Read the model definition and answer for the solid it produces. Units are mm, in the model's axes. Face numbers are marked on the shaded views. A direction names the side the tool comes from. Coordinates: 2 decimals unless noted, no trailing zeros. Loops run counter-clockwise (first coordinate to the right, second up) from the corner with the lowest first, then second, coordinate; pieces in that order, holes last.
from build123d import *

# Parameters (mm, degrees)
F1_DEPTH     = 12.7
F0_W         = 50.8
F0_H         = 7.112
F2_DEPTH     = 25.4
F0_W_2       = 12.7
F0_H_2       = 21.59
F3_DEPTH     = 76.2
F4_DEPTH     = 76.2
F5_SIZE2     = 21.9970452561
F5_SIZE      = 12.7
F6_SIZE2     = 21.9970452561
F6_SIZE      = 12.7
F7_R         = 7.62
F8_T1_DEPTH  = 70.3962243683
F8_T3_DEPTH  = 70.3962243683
F8_T5_DEPTH  = 51.8924487366
F8_T7_DEPTH  = 51.8924487366
F8_T13_DEPTH = 89.9924487366
F8_T17_DEPTH = 89.9924487366


# Not quite as in the source:
# - a fillet or chamfer that OpenCascade refuses, or shapes differently, is made with other operations: its cross-section is extruded or revolved along the edge and cut away or added


with BuildPart() as f1:
    # F0 (on Front) → F1 (new body)
    with BuildSketch(Plane.XZ):
        Polygon((25.4, -14.351), (25.4, 7.239), (12.7, 7.239), (-38.1, 7.239), (-38.1, -14.351), align=None)
    extrude(amount=-F1_DEPTH)

    # F0 (on Front) → F2 (join)
    with BuildSketch(Plane.XZ):
        with Locations((-12.7, 10.795)):
            Rectangle(F0_W, F0_H)
    extrude(amount=-F2_DEPTH)

    # F0 (on Front) → F3 (join)
    with BuildSketch(Plane.XZ):
        with Locations((31.75, -3.556)):
            Rectangle(F0_W_2, F0_H_2)
        with Locations((31.75, 10.795)):
            Rectangle(F0_W_2, F0_H)
    extrude(amount=-F3_DEPTH)

    # F0 (on Front) → F4 (join)
    with BuildSketch(Plane.XZ):
        with Locations((19.05, 10.795)):
            Rectangle(F0_W_2, F0_H)
    extrude(amount=-F4_DEPTH)

    # F5
    f5_edges = [f1.edges().sort_by_distance(p)[0] for p in [
        (38.1, 76.2, 0),
    ]]
    f5_side = f1.faces().sort_by_distance((29.228014, 76.2, 2.143688))[0]
    chamfer(f5_edges, length=F5_SIZE, length2=F5_SIZE2, reference=f5_side)

    # F6
    f6_edges = [f1.edges().sort_by_distance(p)[0] for p in [
        (-38.1, 0, 0),
    ]]
    chamfer(f6_edges, length=F6_SIZE, length2=F6_SIZE2)

    # F7
    f7_edges = [f1.edges().sort_by_distance(p)[0] for p in [
        (38.1, 27.101477, 14.351),
        (10.998523, 0, 14.351),
        (38.1, 0, 0),
    ]]
    fillet(f7_edges, radius=F7_R)

    # F8: chamfer of 7.62 on 4 edges, made by hand

    # F8_s2 → F8_t1 (cut)
    with BuildSketch(Plane.YZ.offset(-57.6962243683)):
        Polygon((17.78, 14.351), (25.4, 6.731), (25.4, 14.351), align=None)
    extrude(amount=F8_T1_DEPTH, mode=Mode.SUBTRACT)

    # F8_s4 → F8_t3 (cut)
    with BuildSketch(Plane.XZ.offset(-95.7962243683)):
        Polygon((20.32, 14.351), (12.7, 6.731), (12.7, 14.351), align=None)
    extrude(amount=F8_T3_DEPTH, mode=Mode.SUBTRACT)

    # F8_s6 → F8_t5 (cut)
    with BuildSketch(Plane.YZ.offset(-6.8962243683)):
        Polygon((68.58, 14.351), (76.2, 6.731), (76.2, 14.351), align=None)
    extrude(amount=F8_T5_DEPTH, mode=Mode.SUBTRACT)

    # F8_s8 → F8_t7 (cut)
    with BuildSketch(Plane.XZ.offset(-44.9962243683)):
        Polygon((-30.48, 14.351), (-38.1, 6.731), (-38.1, 14.351), align=None)
    extrude(amount=F8_T7_DEPTH, mode=Mode.SUBTRACT)


with BuildPart() as f8_tool11:
    # F8_s12 → F8_t13 (new body)
    with BuildSketch(Plane.YZ.offset(32.2962243683)):
        Polygon((17.78, 14.351), (25.4, 6.731), (25.4, 14.351), align=None)
    extrude(amount=-F8_T13_DEPTH)

    split(bisect_by=Plane.YZ.offset(12.7), keep=Keep.TOP)


with BuildPart() as f8_tool15:
    # F8_s16 → F8_t17 (new body)
    with BuildSketch(Plane.XZ.offset(-5.8037756317)):
        Polygon((20.32, 14.351), (12.7, 6.731), (12.7, 14.351), align=None)
    extrude(amount=-F8_T17_DEPTH)

    split(bisect_by=Plane.XZ.offset(-25.4), keep=Keep.TOP)


with BuildPart() as f8_tool11_1:
    add(f8_tool11.part)

    # F8_t19: intersect F8_tool15
    add(f8_tool15.part, mode=Mode.INTERSECT)


with BuildPart() as f1_1:
    add(f1.part)

    # F8_t9: cut F8_tool11
    add(f8_tool11_1.part, mode=Mode.SUBTRACT)


solid = f1_1.part
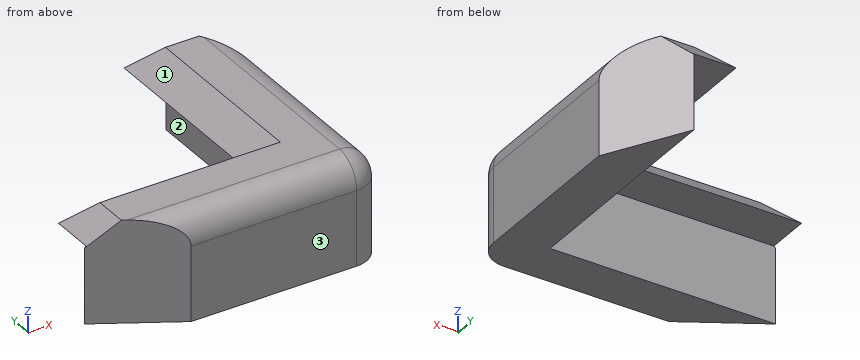
Item 1: Given pin 1 (1.5 mm diameter, centred on y = 63.5, z = 1.5, fed in from -X); pin 2 (6.5 mm diameter, centred on x = 5.5, z = 1, fed in from +Y); pin 3 (12 mm diameter, centred on x = 9.5, y = 41, fed in from +Z), each flat-ended and moving along its own axis, determine where each tip first touches the part or whether it passes through.
Numbers:
pin 1: stops at x = 25.4
pin 2: stops at y = 12.7
pin 3: stops at z = 9.53
Item 2: Which of the six approach directions +Z, -Z, +X, -X, +Y, -Y give full straight-line access (tool end or side, diameter ignored) to the marked faces 1, 2 and 3?
Numbers:
face 1: +Z, -X, +Y
face 2: -Z, -X, +Y
face 3: +Z, -Z, +X, -X, -Y
Item 3: A cutting plane is placed at B-B on z = 3.5. Determine the outline of the cut face in (x, y).
Numbers:
outline: (-38.1, 12.7) - (-16.1, 0) - (30.48, 0) arc R7.62 ccw to (38.1, 7.62) - (38.1, 54.2) - (25.4, 76.2) - (25.4, 12.7) - close
Item 4: A cutting plane is placed at A-A on x = 8. Determine the outline of the cut face in (y, z), then the cut area to 3 significant figures.
Numbers:
outline: (0, -14.35) - (12.7, -14.35) - (12.7, 7.24) - (24.89, 7.24) - (17.78, 14.35) - (7.62, 14.35) arc R7.62 ccw to (0, 6.73) - close
area: 413 mm2
Item 5: Find the intervals of material crossed by line 1 along Y through (x, z) = (2, -11); line 2 along X through (y, z) = (44, 2.75); line 3 along Y through (x, z) = (-18, 5), in increasing order.
Numbers:
line 1: y = 0 to 12.7
line 2: x = 25.4 to 38.1
line 3: y = 1.1 to 12.7
Item 6: A cutting plane is placed at C-C on x = 18. Determine the outline of the cut face in (y, z), then the cut area to 3 significant figures.
Numbers:
outline: (0, -14.35) - (12.7, -14.35) - (12.7, 7.24) - (75.69, 7.24) - (70.9, 12.03) - (20.1, 12.03) - (17.78, 14.35) - (7.62, 14.35) arc R7.62 ccw to (0, 6.73) - close
area: 657 mm2
